from build123d import *

# Parameters (mm, degrees)
F0_W     = 3.689654345
F0_H     = 2
F0_W_2   = 6
F0_H_2   = 6
F0_R     = 1.1
F0_W_3   = 3.6920479782
F0_W_4   = 3.5541171093
F1_DEPTH = 3
F2_R     = 2.99999


# Not quite as in the source:
# - a fillet or chamfer is up to 0.001 mm smaller than in the source, because OpenCascade refuses the exact size


with BuildPart() as f1:
    # F0 (on Front) → F1 (new body)
    with BuildSketch(Plane.XZ):
        with BuildLine():
            Line((25.5162836348, 23.2549019608), (-25.4837163652, 23.2549019608))
            ThreePointArc((-25.4837163652, 23.2549019608), (-27.6050367088, 22.3762223043), (-28.4837163652, 20.2549019608))
            Line((-28.4837163652, 20.2549019608), (-28.4837163652, -14.7450980392))
            ThreePointArc((-28.4837163652, -14.7450980392), (-27.6050367088, -16.8664183828), (-25.4837163652, -17.7450980392))
            Line((-25.4837163652, -17.7450980392), (24.5162836348, -17.7450980392))
            ThreePointArc((24.5162836348, -17.7450980392), (26.6376039783, -16.8664183828), (27.5162836348, -14.7450980392))
            Line((27.5162836348, -14.7450980392), (28.5162836348, 20.2549019608))
            ThreePointArc((28.5162836348, 20.2549019608), (27.6376039783, 22.3762223043), (25.5162836348, 23.2549019608))
        make_face()
        Polygon((-25.4837163652, -8.7450980392), (-25.4837163652, -6.7450980392), (-25.4837163652, -4.7450980392), (-25.4837163652, -2.7450980392), (-25.4837163652, -0.7450980392), (-25.4837163652, 14.2549019608), (-25.4837163652, 20.2549019608), (-19.4837163652, 20.2549019608), (19.5162836348, 20.2549019608), (25.5162836348, 20.2549019608), (25.5162836348, 14.2549019608), (25.5162836348, -14.7450980392), (24.5162836348, -14.7450980392), (18.5162836348, -14.7450980392), (-19.4837163652, -14.7450980392), (-25.4837163652, -14.7450980392), align=None, mode=Mode.SUBTRACT)
        Polygon((-21.929599256, -6.7450980392), (-25.4837163652, -6.7450980392), (-25.4837163652, -8.7450980392), (-19.4837163652, -8.7450980392), (-19.4837163652, -14.7450980392), (18.5162836348, -14.7450980392), (18.5162836348, -8.7450980392), (24.5162836348, -8.7450980392), (24.5162836348, -14.7450980392), (25.5162836348, -14.7450980392), (25.5162836348, 14.2549019608), (19.5162836348, 14.2549019608), (19.5162836348, 20.2549019608), (-19.4837163652, 20.2549019608), (-19.4837163652, 14.2549019608), (-25.4837163652, 14.2549019608), (-25.4837163652, -0.7450980392), (-21.791668387, -0.7450980392), (-21.791668387, -2.7450980392), (-25.4837163652, -2.7450980392), (-25.4837163652, -4.7450980392), (-21.929599256, -4.7450980392), align=None)
        with Locations((22.6714564623, -1.7450980392)):
            Rectangle(F0_W, F0_H, mode=Mode.SUBTRACT)
        with Locations((22.5162836348, 17.2549019608)):
            Rectangle(F0_W_2, F0_H_2)
        with Locations((22.5162836348, 17.2549019608)):
            Circle(F0_R, mode=Mode.SUBTRACT)
        with Locations((-22.4837163652, 17.2549019608)):
            Rectangle(F0_W_2, F0_H_2)
        with Locations((-22.4837163652, 17.2549019608)):
            Circle(F0_R, mode=Mode.SUBTRACT)
        with Locations((-22.4837163652, -11.7450980392)):
            Rectangle(F0_W_2, F0_H_2)
        with Locations((-22.4837163652, -11.7450980392)):
            Circle(F0_R, mode=Mode.SUBTRACT)
        with Locations((21.5162836348, -11.7450980392)):
            Rectangle(F0_W_2, F0_H_2)
        with Locations((21.5162836348, -11.7450980392)):
            Circle(F0_R, mode=Mode.SUBTRACT)
        with Locations((-23.6376923761, -1.7450980392)):
            Rectangle(F0_W_3, F0_H)
        with Locations((22.6714564623, -1.7450980392)):
            Rectangle(F0_W, F0_H)
        with Locations((-23.7066578106, -5.7450980392)):
            Rectangle(F0_W_4, F0_H)
    extrude(amount=F1_DEPTH)

    # F2 (radius 3 in the source; OpenCascade refuses exactly that, so slightly less here)
    f2_edges = [f1.edges().sort_by_distance(p)[0] for p in [
        (-23.583716, -3, -11.745098),
        (-23.583716, -3, 17.254902),
        (21.416284, -3, 17.254902),
        (20.416284, -3, -11.745098),
    ]]
    fillet(f2_edges, radius=F2_R)


solid = f1.part
Geometry check sheet. Reference: the model listing, model coordinates, mm. Round coordinates to 2 decimals unless told otherwise and drop trailing zeros. Loops run counter-clockwise (first coordinate to the right, second up) from the corner with the lowest first, then second, coordinate; pieces in that order, holes last.
Item 1: Cross-section at A-A on y = -1.4. Record the boundary of the cut face in (x, z).
Item 2: Thickness scan on line 1 (Z direction, x = 22, y = -2.4); line 2 (Z direction, x = 23.5, y = -0.4); line 3 (Z direction, x = 23, y = -0.05). Record the ranges inside material, lowest first.
Item 3: Cross-section at B-B on x = -23. Count the separate pieces of the cut face and the enclosed holes in it, then the cut area to 3 significant figures.
Answer sheet:
1. outline: (-28.48, -14.75) arc R3 ccw to (-25.48, -17.75) - (24.52, -17.75) arc R3 ccw to (27.52, -14.75) - (28.52, 20.25) arc R3 ccw to (25.52, 23.25) - (-25.48, 23.25) arc R3 ccw to (-28.48, 20.25) - close; hole circle Ø2.89 at (-22.48, -11.75); hole circle Ø2.89 at (-22.48, 17.25); hole circle Ø2.89 at (21.52, -11.75); hole circle Ø2.89 at (22.52, 17.25)
2. line 1: z = -17.75 to -13.99, -9.5 to 15.01, 19.5 to 23.25
2. line 2: z = -17.75 to 16.71, 17.8 to 23.25
2. line 3: z = -17.75 to 16.27, 18.24 to 23.25
3. separate pieces: 3
3. enclosed holes: 0
3. area: 103 mm2
